Autodesk Inventor part; units mm, degrees
ref_plane "YZ Plane" through (0, 0, 0) normal (1, 0, 0) x (0, 1, 0)
ref_plane "XZ Plane" through (0, 0, 0) normal (0, 1, 0) x (-1, 0, 0)
ref_plane "XY Plane" through (0, 0, 0) normal (0, 0, 1) x (1, 0, 0)
sketch "Sketch1" plane through (0, 0, 0) normal (0, 1, 0) x (-1, 0, 0)
  line L0 (11, -16) -> (-11, -16)
  line L1 (-11, -16) -> (-11, 16)
  line L2 (-11, 16) -> (11, 16)
  line L3 (11, 16) -> (11, -16)
  line L4 (11, -16) -> (-11, 16) construction
  line L5 (-11, -16) -> (11, 16) construction
  circle A0 centre (-2, 6.5) radius 4.8
  line L6 (-2, 6.5) -> (-2, -6.5)
  circle A1 centre (-2, -6.5) radius 4.8
  line L7 (-2, 11.3) -> (-11, 11.3)
  line L8 (-2, 1.7) -> (-11, 1.7)
  line L9 (-2, -1.7) -> (-11, -1.7)
  line L10 (-2, -11.3) -> (-11, -11.3)
  point P0 (0, 0)
  point P1 (-2, 0)
  dimension "d0" = 22
  dimension "d1" = 32
  dimension "d2" = 9.6
  dimension "d3" = 13
  dimension "d4" = 9.6
extrude "Extrusion1" add sketch "Sketch1" along normal blind 2 contours L0 L1 L10 A1 L6 A0 L7 L2 L3 | L1 L8 L6 L9
sketch "Sketch2" plane through (0, 0, 0) normal (0, -1, 0) x (1, 0, 0)
  line L0 (-11, 16) -> (11, 16)
  line L1 (11, 16) -> (-11, 16)
  line L2 (-11, -16) -> (-11, 16)
  line L3 (-11, 16) -> (-11, -16)
  line L4 (11, -16) -> (-11, -16)
  line L5 (-11, -16) -> (11, -16)
  line L6 (11, -16) -> (11, -14)
  line L7 (11, -11.3) -> (11, -16)
  line L8 (11, -14) -> (-5, -14)
  line L9 (-5, -14) -> (-5, 14)
  line L10 (-5, 14) -> (11, 14)
  line L11 (11, 16) -> (11, 11.3)
  point P0 (0, 0)
  dimension "d7" = 2
  dimension "d8" = 16
  dimension "d9" = 28
extrude "Extrusion2" add sketch "Sketch2" along normal blind 2.75
sketch "Sketch3" plane through (-11, 2, -16) normal (-1, 0, 0) x (0, 0, 1)
  line L0 (0, 0) -> (0, -4.75)
  line L1 (0, -4.75) -> (32, -4.75)
  line L2 (32, -4.75) -> (32, 49.75)
  line L3 (32, 49.75) -> (0, 49.75)
  line L4 (0, 49.75) -> (0, -4.75)
  point P0 (16, -2)
  dimension "d12" = 54.5
extrude "Extrusion3" add sketch "Sketch3" along normal blind 3
sketch "Sketch4" plane through (0, -2.75, 0) normal (0, -1, 0) x (1, 0, 0)
  line L0 (11, 16) -> (11, 11.3)
  line L1 (11, 16) -> (-39, 16)
  line L2 (-39, 16) -> (-39, -16)
  line L3 (-39, -16) -> (11, -16)
  line L4 (11, -16) -> (11, 16)
  point P0 (0, 0)
  dimension "d15" = 50
extrude "Extrusion4" add sketch "Sketch4" along normal blind 2
sketch "Sketch5" plane through (-5, 0, 14) normal (1, 0, 0) x (0, 0, -1)
  line L0 (0, 0) -> (0, -2.75)
  line L1 (30, -2.75) -> (-2, -2.75)
  line L2 (0, 0) -> (2.9896, 0)
  line L3 (2.9896, 0) -> (2.9896, -2.75)
  line L4 (2.9896, -2.75) -> (0, -2.5)
  line L5 (0, -2.5) -> (0, 0)
  point P0 (14, 0)
  dimension "d18" = 3
extrude "Extrusion5" cut sketch "Sketch5" against normal up to surface (9 mm away)
sketch "Sketch6" plane through (11, 0, 1.7) normal (1, 0, 0) x (0, 0, -1)
  line L0 (0, 0) -> (0, 2)
  line L1 (3.4, 0) -> (3.4, 2)
  line L2 (0, 1) -> (3.4, 1)
  line L3 (3.4, 1) -> (3.4, 2)
  line L4 (3.4, 2) -> (0, 2)
  line L5 (0, 2) -> (0, 1)
  point P0 (1.7, 0)
extrude "Extrusion6" cut sketch "Sketch6" against normal blind 2.2
sketch "Sketch8" plane through (-14, 2, -16) normal (-1, 0, 0) x (0, 0, 1)
  circle A0 centre (24.6, 39.75) radius 2.75
  circle A1 centre (24.6, 39.75) radius 1.4
  line L0 (4, 47.25) -> (28, 47.25) construction
  line L1 (28, 47.25) -> (28, -1.75) construction
  line L2 (28, -1.75) -> (4, -1.75) construction
  line L3 (4, -1.75) -> (4, 47.25) construction
  circle A2 centre (7.4, 5.75) radius 2.75
  circle A3 centre (7.4, 5.75) radius 1.4
  line L4 (4, 47.25) -> (28, -1.75) construction
  line L5 (32, -4.75) -> (32, -6.75) construction
  line L6 (32, 49.75) -> (0, 49.75) construction
  line L7 (0, -4.75) -> (32, 49.75) construction
  point P0 (16, -2)
  point P1 (16, 22.75)
  point P2 (16, 22.5)
  dimension "d24" = 5.5
  dimension "d25" = 2.8
  dimension "d26" = 24
  dimension "d27" = 49
  dimension "d28" = 3.4
  dimension "d29" = 7.5
  dimension "d30" = 5.5
  dimension "d31" = 2.8
  dimension "d32" = 3.4
  dimension "d33" = 7.5
extrude "Extrusion7" add sketch "Sketch8" along normal blind 5
sketch "Sketch9" plane through (0, 0, 0) normal (0, 0, 1) x (1, 0, 0)
  line L0 (-14, -2.75) -> (-14, 51.75)
  line L1 (-12.5, 56.75) -> (-12.5, 54.25) construction
  line L2 (-12.25, 56.75) -> (-12.25, 54.25)
  line L3 (-12.25, 54.25) -> (-12.75, 54.25)
  line L4 (-12.75, 54.25) -> (-12.75, 56.75)
  line L5 (-12.75, 56.75) -> (-12.25, 54.25) construction
  line L6 (-12.25, 56.75) -> (-12.75, 54.25) construction
  circle A0 centre (-12.5, 63.45) radius 6.7
  line L7 (-12.5, 63.45) -> (-12.5, 56.75) construction
  line L8 (-12.25, 56.75) -> (-12.25, 59.7585)
  line L9 (-12.75, 59.7585) -> (-12.75, 56.75)
  line L10 (-12.25, 59.7585) -> (-12.25, 70.1453)
  line L11 (-12.25, 70.1453) -> (-12.75, 70.1453)
  line L12 (-12.75, 70.1453) -> (-12.75, 59.7585)
  line L13 (-12.5, 63.45) -> (-5.8, 63.45) construction
  line L14 (-12.5, 63.45) -> (-5.8, 63.45) construction
  line L15 (-11, 51.75) -> (-14, 51.75)
  line L16 (-14, 51.75) -> (-11, 51.75)
  line L17 (-11, 51.75) -> (-11, 56.75)
  line L18 (-11, 56.75) -> (-14, 56.75)
  line L19 (-14, 56.75) -> (-14, 51.75)
  line L20 (-14, 56.75) -> (-11, 56.75)
  line L21 (-11, 56.75) -> (-11, 56.9201)
  line L22 (-11, 56.9201) -> (-14, 56.9201)
  line L23 (-14, 56.9201) -> (-14, 56.75)
  circle A1 centre (-12.5, 63.45) radius 3.5
  line L24 (-12.5, 63.45) -> (-5.8, 63.45) construction
  line L25 (-12.5, 63.45) -> (-5.8, 63.45) construction
  circle A2 centre (-16.1062, 67.0562) radius 1.6
  circle A3 centre (-8.8938, 67.0562) radius 1.6
  point P0 (0, 0)
  point P1 (-12.5, 55.5)
  point P2 (-12.75, 56.7547)
  point P3 (-12.25, 56.7547)
  point P4 (-17.2376, 68.1876)
  point P5 (-12.75, 59.9589)
  point P6 (-14.9749, 65.9249)
  point P7 (-10.0251, 65.9249)
  point P8 (-12.25, 59.9589)
  point P9 (-7.7624, 68.1876)
  dimension "d47" = 0.5
  dimension "d49" = 13.4
  dimension "d50" = 5
  dimension "d57" = 7
extrude "Extrusion8" add sketch "Sketch9" along normal mid plane 32 contours L18 L17 L15 L19 L4 L3 L2 | L8 A0 L21 L18 | L8 L22 A0 | L22 L8 L10 A1 A3 A0 | L9 L18 L23 A0 | A0 L22 L9 | L22 A0 A2 A1 L12 L9 | A3 | A2
sketch "Sketch10" plane through (-11, 2, 16) normal (0, 0, 1) x (1, 0, 0)
  line L0 (-1.75, 52.25) -> (-1.25, 52.25)
  line L1 (-1.75, 52.25) -> (-1.25, 52.25)
  line L2 (-1.25, 52.25) -> (-1.25, 37.25)
  line L3 (-1.25, 37.25) -> (-1.75, 37.25)
  line L4 (-1.75, 37.25) -> (-1.75, 52.25)
  line L5 (-1.75, 37.25) -> (-2.4777, 58.0893)
  arc A0 (-3.9749, 63.9249) -> (-1.75, 57.9589) centre (-1.5, 61.45) ccw
  line L6 (-1.75, 37.25) -> (19.102, 37.25) construction
  line L7 (-1.25, 37.25) -> (-0.5223, 58.0893)
  arc A1 (-1.25, 57.9589) -> (0.9749, 63.9249) centre (-1.5, 61.45) ccw
  line L8 (-1.25, 37.25) -> (19.602, 37.25) construction
  arc A2 (-2.4777, 58.0893) -> (-0.5223, 58.0893) centre (-1.5, 61.45) ccw
  point P0 (11, -2)
  dimension "d51" = 15
  dimension "d60" = 92
  dimension "d61" = 88
extrude "Extrusion9" cut sketch "Sketch10" against normal through all contours L0 L2 L3 L4
sketch "Sketch11" plane through (0, 0, 0) normal (0, 0, 1) x (1, 0, 0)
  line L0 (-14, -2.75) -> (-14, 56.9201)
  line L1 (-12.5, 63.45) -> (-18.3024, 60.1)
  line L2 (-14, 56.9201) -> (-14, 62.9804)
  circle A0 centre (-12.5, 63.45) radius 6.7
  point P0 (0, 0)
  point P1 (-14, 62.584)
extrude "Extrusion10" cut sketch "Sketch11" along normal mid plane 10 contours L2 A0 L1 picked at (-14.4333, 58.9557)
sketch "Sketch13" plane through (0, 2, 0) normal (0, 1, 0) x (1, 0, 0)
  line L0 (-11, 16) -> (-11, -16)
  line L1 (-11, 0) -> (-9, 0) construction
  line L2 (-11, 4.5) -> (-7, 4.5)
  line L3 (-7, 4.5) -> (-7, -4.5)
  line L4 (-7, -4.5) -> (-11, -4.5)
  line L5 (-11, -4.5) -> (-11, 4.5)
  line L6 (-11, 4.5) -> (-7, -4.5) construction
  line L7 (-7, 4.5) -> (-11, -4.5) construction
  point P0 (0, 0)
  point P1 (-11, -4.5)
  dimension "d66" = 2
  dimension "d67" = 4
  dimension "d68" = 9
extrude "Extrusion12" add sketch "Sketch13" along normal up to surface
sketch "Sketch12" plane through (-14, 2, -16) normal (-1, 0, 0) x (0, 0, 1)
  line L0 (0, 54.9201) -> (32, 54.9201)
  line L1 (16, 54.9201) -> (16, 50.9201) construction
  circle A0 centre (16, 50.9201) radius 1.5
  point P0 (16, -2)
  dimension "d62" = 4
  dimension "d63" = 3
extrude "Extrusion11" cut sketch "Sketch12" against normal through all
sketch "Sketch14" plane through (-7, 2, 4.5) normal (1, 0, 0) x (0, 0, -1)
  line L0 (7.4, 49.2458) -> (4.5, 47.5714)
  line L1 (4.5, 47.5714) -> (1.6, 49.2458)
  line L2 (1.6, 49.2458) -> (1.6, 52.5944)
  line L3 (1.6, 52.5944) -> (4.5, 54.2687)
  line L4 (4.5, 54.2687) -> (7.4, 52.5944)
  line L5 (7.4, 52.5944) -> (7.4, 49.2458)
  circle A0 centre (4.5, 50.9201) radius 1.5
  point P0 (4.5, -2)
  point P1 (4.5, 50.9201)
  dimension "d71" = 5.8
  dimension "d74" = 0
extrude "Extrusion13" cut sketch "Sketch14" against normal blind 2.5
properties part number "prototype_8_1_3DPrint"
The listing builds one solid part. Answer for the finished solid, in the listing's coordinates (mm). A direction names the side the tool comes from. Coordinates: 2 decimals unless noted, no trailing zeros. Loops run counter-clockwise (first coordinate to the right, second up) from the corner with the lowest first, then second, coordinate; pieces in that order, holes last. Notation, with made-up numbers: M 33.5,30 L 39.5,30 A23 ccw 39.5,40 Z; hole C -0.5,41 d5. An arc over 180 degrees is marked long. Answer in a Markdown table with one row per item.
1) Find section D-D (y = 38). Determine the outline of the cut face in (x, z).
Answers below:
| item | result |
|---|---|
| outline | M -14,-16 L -11,-16 L -11,-4.5 L -7,-4.5 L -7,4.5 L -11,4.5 L -11,16 L -14,16 Z |
2) Determine the mould class of faces 1 (the flat face through (-12, 16, -16)), 2 (the cylindrical face through (-16.46, 8.8, -6.06)), 3 (the cylindrical face through (-10.894, 51.456, -0.325)) for opening direction Z: released by +Z, released by -Z, zero draft, split by the parting line, or undercut.
Answers below:
| item | result |
|---|---|
| face 1 | released by -Z |
| face 2 | split by the parting line |
| face 3 | undercut |
3) Find the intervals of material crossed by probe 1 along X at (y, z) = (50.5, 10); probe 2 along Y at (x, z) = (4, 1.5); probe 3 along Y at (x, z) = (-10, -8.5), in increasing order.
Answers below:
| item | result |
|---|---|
| probe 1 | -14 to -12.75, -12.25 to -11 |
| probe 2 | -4.75 to -2.75, 0 to 2 |
| probe 3 | -4.75 to 2, 57.23 to 61, 65.9 to 68.21 |
4) Find section A-A (x = -0.5). Determine the outline of the cut face in (y, z).
Answers below:
| item | result |
|---|---|
| outline | M -4.75,-16 L 2,-16 L 2,-10.6 L 0,-10.6 L 0,-14 L -2.75,-14 L -2.75,14 L 0,14 L 0,10.6 L 2,10.6 L 2,16 L -4.75,16 Z; M 0,-2.4 L 2,-2.4 L 2,2.4 L 0,2.4 Z |
5) Find section C-C (z = -8). Determine the outline of the cut face in (x, y), then the cut area to 3 significant figures.
Answers below:
| item | result |
|---|---|
| outline | M -39,-4.75 L 11,-4.75 L 11,-2.75 L -5,-2.75 L -5,0 L -2.56,0 L -2.56,2 L -11,2 L -11,56.92 A6.7 ccw -7.76,68.19 A1.6 ccw -10.03,65.92 A3.5 cw -12.25,59.96 L -12.25,39.25 L -12.75,39.25 L -12.75,59.96 A3.5 cw -14.97,65.92 A1.6 ccw -17.24,68.19 A6.7 ccw -14,56.92 L -14,10.43 L -19,10.43 L -19,9.01 L -14,9.01 L -14,6.49 L -19,6.49 L -19,5.07 L -14,5.07 L -14,-2.75 L -39,-2.75 Z |
| area | 401 mm^2 |
6) Which of the six approach directions +Z, -Z, +X, -X, +Y, -Y give full straight-line access (tool end or side, diameter ignored) to faces 4 (the flat face through (-8.23, 55.42, 1.47)), 5 (the flat face through (-2, -1, 14)), 6 (the flat face through (-12.25, 50, 0))?
Answers below:
| item | result |
|---|---|
| face 4 | +X |
| face 5 | +X, -X |
| face 6 | +Z, -Z, +Y |
7) Given pin 1 (1.4 mm diameter, centred on y = 41.5, z = 8, fed in from -X); pin 2 (6 mm diameter, centred on y = 7.5, z = -9, fed in from -X); pin 3 (3 mm diameter, centred on y = 51.5, z = 0.5, fed in from +X); pin 4 (12 mm diameter, centred on x = -9.5, z = 0.5, fed in from +Y), each flat-ended and moving along its own axis, determine where each tip first touches the part or whether it passes through.
Answers below:
| item | result |
|---|---|
| pin 1 | x = -14 |
| pin 2 | x = -19 |
| pin 3 | x = -7 |
| pin 4 | y = 68.66 |
8) Find section B-B (y = 55.5). Determine the outline of the cut face in (x, z).
Answers below:
| item | result |
|---|---|
| outline | M -14,-16 L -12.75,-16 L -12.75,16 L -14,16 Z; M -12.25,-16 L -11,-16 L -11,-4.5 L -7,-4.5 L -7,-1.33 L -9.5,-1.33 L -9.5,1.33 L -7,1.33 L -7,4.5 L -11,4.5 L -11,16 L -12.25,16 Z |
